Source: CAD feature listing. Evaluate the final solid. Frame: model axes, mm. Face numbers are marked on the shaded views. A direction names the side the tool comes from. Round coordinates to 2 decimals unless told otherwise and drop trailing zeros. Write each loop counter-clockwise with the first axis right and the second up, starting at its lowest first coordinate (ties: lowest second). Pieces come first, ordered by that corner, then holes. Notation, with made-up numbers: M 37,68 L 85,68 A15 cw 85,79 Z; hole C 84,14.25 d10. An arc over 180 degrees is marked long. Answer in a Markdown table with one row per item.
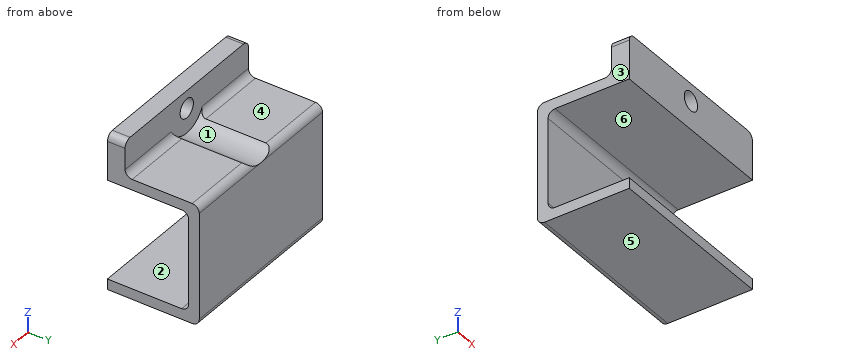
Autodesk Inventor part; units mm, degrees
ref_plane "YZ Plane" through (0, 0, 0) normal (1, 0, 0) x (0, 1, 0)
ref_plane "XZ Plane" through (0, 0, 0) normal (0, 1, 0) x (-1, 0, 0)
ref_plane "XY Plane" through (0, 0, 0) normal (0, 0, 1) x (1, 0, 0)
sketch "Esquisse1" plane through (0, 0, 0) normal (0, 1, 0) x (-1, 0, 0)
  line L0 (-12.5, 11) -> (12.5, 11)
  line L1 (12.5, 11) -> (12.5, -11)
  line L2 (12.5, -11) -> (-12.5, -11)
  line L3 (-12.5, -11) -> (-12.5, 11)
  point P0 (0, 0)
  dimension "d0" = 25
  dimension "d1" = 22
  dimension "d2" = 11
  dimension "d3" = 12.5
extrude "Extrusion1" add sketch "Esquisse1" along normal blind 13
sketch "Esquisse2" plane through (0, 13, 0) normal (0, 1, 0) x (1, 0, 0)
  line L0 (-12.5, 11) -> (-12.5, -11)
  line L1 (-12.5, -6) -> (12.5, -6)
  line L2 (12.5, -6) -> (12.5, -11)
  line L3 (12.5, -11) -> (-12.5, -11)
  line L4 (-12.5, -11) -> (-12.5, -6)
  point P0 (0, 0)
  dimension "d6" = 5
extrude "Extrusion3" cut sketch "Esquisse2" against normal blind 10.5
fillet "Congé2" radius 1 1 edges at (0, 2.5, 6)
sketch "Esquisse4" plane through (0, 13, 0) normal (0, 1, 0) x (1, 0, 0)
  circle A0 centre (0, -8.5) radius 3.5
  line L0 (12.5, -11) -> (-12.5, -11)
  point P0 (12.5, -6)
  point P1 (0, 0)
  dimension "d11" = 7
  dimension "d12" = 2.5
  dimension "d13" = 5
extrude "Extrusion4" cut sketch "Esquisse4" against normal blind 10.5
sketch "Esquisse6" plane through (0, 0, 0) normal (0, -1, 0) x (1, 0, 0)
  line L0 (-12.5, 11) -> (-12.5, -11)
  line L1 (-12.5, -11) -> (12.5, -11)
  line L2 (12.5, -11) -> (12.5, 11)
  line L3 (-12.5, -9.5) -> (12.5, -9.5)
  line L4 (12.5, -9.5) -> (12.5, 4.5)
  line L5 (12.5, 4.5) -> (-12.5, 4.5)
  line L6 (-12.5, 4.5) -> (-12.5, -9.5)
  point P0 (0, 0)
  dimension "d17" = 0
  dimension "d18" = 0
  dimension "d19" = 1.5
  dimension "d20" = 6.5
extrude "Extrusion5" cut sketch "Esquisse6" against normal blind 11.5 contours L5 L2 L3 L0
fillet "Congé3" radius 1 2 edges at (-12.5, 1.25, 11) (12.5, 1.25, 11)
fillet "Congé4" radius 1 5 edges at (0, 11.5, -9.5) (0, 13, -11) (0, 11.5, 4.5) (-7.4747, 13, 6) (7.4747, 13, 6)
sketch "Esquisse7" plane through (0, 2.5, 0) normal (0, 1, 0) x (1, 0, 0)
  arc A0 (3.1623, -7) -> (-3.1623, -7) centre (0, -8.5) ccw
  circle A1 centre (0, -8.5) radius 1.35
  point P0 (0, 0)
  dimension "d27" = 2.7
extrude "Extrusion6" cut sketch "Esquisse7" against normal through all
equation "\"d12\" = 0.5 * d13"
properties part number "capot" material "Plastique ABS"
Q1. Section B-B (z = 8.5). Return loops of the section in (x, y), and give its area (4 significant figures).
Solutions:
| item | result |
|---|---|
| outline | M -12.5,0 L -1.35,0 L -1.35,2.5 L -12.5,2.5 Z; M 1.35,0 L 12.5,0 L 12.5,2.5 L 1.35,2.5 Z |
| area | 55.75 mm2 |
Q2. Access query for the marked faces 4, 5 and 6. Directions: +Z, -Z, +X, -X, +Y, -Y. A direction counts if a zero-diameter tool reaches every point of the face in a straight line with its end or side. Return the directions, or none.
Solutions:
| item | result |
|---|---|
| face 4 | +Z, +X, -X, +Y |
| face 5 | -Z, +X, -X, +Y, -Y |
| face 6 | +X, -X, -Y |
Q3. Section D-D (x = -4.75). Return loops of the section in (y, z), and give its area (3 significant figures).
Solutions:
| item | result |
|---|---|
| outline | M 0,-11 L 12,-11 A1 ccw 13,-10 L 13,5 A1 ccw 12,6 L 3.5,6 A1 cw 2.5,7 L 2.5,11 L 0,11 L 0,4.5 L 10.5,4.5 A1 cw 11.5,3.5 L 11.5,-8.5 A1 cw 10.5,-9.5 L 0,-9.5 Z |
| area | 72.7 mm2 |
Q4. Contact query for flat-ended pins moving along their axis: pin 1 Ø3.5 at (x, z) = (-4.5, -5) entering from -Y; pin 2 Ø7 at (x, y) = (7, 9) entering from +Z; pin 3 Ø4.5 at (x, z) = (0, 8.5) entering from +Y. Output: stop coordinate, or through.
Solutions:
| item | result |
|---|---|
| pin 1 | stops at y = 11.5 |
| pin 2 | stops at z = 6 |
| pin 3 | stops at y = 2.5 |
Q5. Material intervals for probe 1 along Z at (x, y) = (0, 1); probe 2 along X at (y, z) = (0.7, 8.5); probe 3 along Z at (x, y) = (4, 7.5), sorted ascending.
Solutions:
| item | result |
|---|---|
| probe 1 | z = -11 to -9.5, 4.5 to 7.15, 9.85 to 11 |
| probe 2 | x = -12.5 to -1.35, 1.35 to 12.5 |
| probe 3 | z = -11 to -9.5, 4.5 to 6 |
Q6. Section C-C (y = 1.5). Return loops of the section in (x, z), and give its area (3 significant figures).
Solutions:
| item | result |
|---|---|
| outline | M -12.5,-11 L 12.5,-11 L 12.5,-9.5 L -12.5,-9.5 Z; M -12.5,4.5 L 12.5,4.5 L 12.5,10 A1 ccw 11.5,11 L -11.5,11 A1 ccw -12.5,10 Z; hole C 0,8.5 d2.7 |
| area | 194 mm2 |
Q7. Section A-A (y = 6.5). Return loops of the section in (x, z), and give its area (3 significant figures).
Solutions:
| item | result |
|---|---|
| outline | M -12.5,-11 L 12.5,-11 L 12.5,-9.5 L -12.5,-9.5 Z; M -12.5,4.5 L 12.5,4.5 L 12.5,6 L 2.45,6 A3.5 cw -2.45,6 L -12.5,6 Z |
| area | 71.6 mm2 |
Q8. Pull-direction query (X, two-part tool) for the marked faces 1, 2 and 3; classes: pulls with the +X half, pulls with the -X half, needs draft (parallel to the pull), parting line crosses it, or undercut.
Solutions:
| item | result |
|---|---|
| face 1 | undercut |
| face 2 | needs draft |
| face 3 | pulls with the -X half |
